Check sheet for the modelled part. Datum: model origin and axes. Units: mm. Coordinates: 2 decimals unless noted, no trailing zeros. Loops run counter-clockwise (first coordinate to the right, second up) from the corner with the lowest first, then second, coordinate; pieces in that order, holes last. Notation, with made-up numbers: (52.25, 30.25) - (87.25, 30.25) arc R31 cw to (87.25, 69.25) - close; hole circle Ø3 at (-19, 12.25). An arc over 180 degrees is marked (long way). Write each question's results on one line, items separated by ' | '. Start each with the question number.
1. Cross-section at C-C (z = -2). Record the cut outline in (x, y).
2. Draft check along X on faces 1 (the face through (71.71, 1.52, 1.26)), 2 (the face through (-1, 0, -1)), 3 (the face through (35.11, 1.48, -43.66)), 4 (the face through (-26.368, 1.479, -54.906)). Enter one of: released by +X, released by -X, zero draft, split by the parting line, or undercut.
3. Thickness scan on line 1 (X direction, y = 1.3, z = -73.5); line 2 (Z direction, x = 35, y = 1.55); line 3 (X direction, y = 2, z = -74). Record the ranges inside material, lowest first. Write a range as [from, to].
4. Cross-section at A-A (y = 1.9). Give the number of separate pieces and of enclosed holes in the cut face, and give its area (3 significant figures).
5. Cross-section at B-B (x = -49). Record the cut outline in (y, z), and give its area (3 significant figures).
6. Gauge pin test, flat ends, axial feed: P1, Ø1.5, axis at x = -41, y = 1, coming from the -Z side; P2, Ø8, axis at x = -2.11, z = -75.5, coming from the +Y side; P3, Ø1.5, axis at y = 1.5, z = -81.5, coming from the -X side; P4, Ø1.5, axis at x = -29.5, y = 1, coming from the +Z side. Record the tip position at first contact, or that the pin passes through.
```python
from build123d import *

# Parameters (mm, degrees)
ESQUISSE1_R             = 2.25
ESQUISSE1_R_2           = 2.5
ESQUISSE1_W             = 6
ESQUISSE1_H             = 10
ESQUISSE1_R_3           = 2.500458525
BOSS_EXTRU_1_DEPTH      = 3
ENL_V_MAT_EXTRU_2_DEPTH = 216


with BuildPart() as part:
    # Esquisse1 → Boss.-Extru.1 (new body)
    with BuildSketch(Plane(origin=(0, 0, 0), x_dir=(1, 0, 0), z_dir=(0, 1, 0))):
        Polygon((-15, -90), (75, -90), (75, 90), (-15, 90), (-15, 70), (-75, 70), (-75, -70), (-15, -70), align=None)
        with Locations(Location((-72.531396859, -50.020890538, 0), (0, 0, 270))):
            Circle(ESQUISSE1_R, mode=Mode.SUBTRACT)
        with Locations(Location((-2.161539128, -75.5, 0), (0, 0, 270))):
            Circle(ESQUISSE1_R_2, mode=Mode.SUBTRACT)
        with Locations(Location((-28.276866627, -56.270890538, 0), (0, 0, 270))):
            Circle(ESQUISSE1_R_2, mode=Mode.SUBTRACT)
        with Locations(Location((-2.161539128, -55.5, 0), (0, 0, 270))):
            Circle(ESQUISSE1_R_2, mode=Mode.SUBTRACT)
        with Locations(Location((-28.276866627, -43.770890538, 0), (0, 0, 270))):
            Circle(ESQUISSE1_R_2, mode=Mode.SUBTRACT)
        with Locations((33, -70)):
            Rectangle(ESQUISSE1_W, ESQUISSE1_H, mode=Mode.SUBTRACT)
        with Locations(Location((28.039441899, -45, 0), (0, 0, 270))):
            Circle(ESQUISSE1_R_3, mode=Mode.SUBTRACT)
        with Locations(Location((-28.476498774, 43.75, 0), (0, 0, 270))):
            Circle(ESQUISSE1_R_2, mode=Mode.SUBTRACT)
        with Locations(Location((-72.731029006, 50, 0), (0, 0, 270))):
            Circle(ESQUISSE1_R, mode=Mode.SUBTRACT)
        with Locations(Location((-28.476498774, 56.25, 0), (0, 0, 270))):
            Circle(ESQUISSE1_R_2, mode=Mode.SUBTRACT)
        with Locations(Location((-2.111629991, 55.5, 0), (0, 0, 270))):
            Circle(ESQUISSE1_R_2, mode=Mode.SUBTRACT)
        with Locations(Location((-2.111629991, 75.5, 0), (0, 0, 270))):
            Circle(ESQUISSE1_R_2, mode=Mode.SUBTRACT)
        with Locations(Location((33, 45, 0), (0, 0, 270))):
            Circle(ESQUISSE1_R_2, mode=Mode.SUBTRACT)
        with Locations((33, 70)):
            Rectangle(ESQUISSE1_W, ESQUISSE1_H, mode=Mode.SUBTRACT)
    extrude(amount=BOSS_EXTRU_1_DEPTH)

    # Esquisse4 → Enlèv. mat.-Extru.2 (cut)
    with BuildSketch(Plane.XY.offset(90)):
        Polygon((68.505970044, 3), (75, 0), (83.303291845, 0), (76.039441899, 3), align=None)
    extrude(amount=-ENL_V_MAT_EXTRU_2_DEPTH, mode=Mode.SUBTRACT)


solid = part.part
```
Established:
1) outline: (-75, 0) - (75, 0) - (68.51, 3) - (-75, 3) - close
2) face 1: released by +X | face 2: zero draft | face 3: undercut | face 4: undercut
3) line 1: [-15, -3.61], [-0.61, 30], [36, 72.19] | line 2: [-90, -75], [-65, -46.5], [-43.5, 65], [75, 90] | line 3: [-15, -4.11], [-0.11, 30], [36, 70.67]
4) separate pieces: 1 | enclosed holes: 14 | area: 23,500 mm^2
5) outline: (0, -70) - (3, -70) - (3, 70) - (0, 70) - close | area: 420 mm^2
6) P1: z = -70 | P2: y = 3 | P3: x = -15 | P4: z = 70
